Print and shaded views of the part. All mm, measured from the part's lowest x, y and z. A direction names the side the tool comes from. Coordinates: 2 decimals unless noted, no trailing zeros. Loops run counter-clockwise (first coordinate to the right, second up) from the corner with the lowest first, then second, coordinate; pieces in that order, holes last.
1) Pin check, flat tips, straight feed: pin 1 Ø1.7 at (y, z) = (16.5, 6.5) entering from +X; pin 2 Ø1.5 at (x, y) = (13, 12) entering from +Z; pin 3 Ø4.5 at (x, z) = (11, 11.5) entering from +Y; pin 4 Ø3 at (y, z) = (17.5, 6.5) entering from -X. Stop position of each tip, or through.
2) Which spindle directions (+Z, -Z, +X, -X, +Y, -Y) get a long thin tool onto all of the face, cutting with end or side? Do the marked faces 1, 2 and 3. Say none if no direction does.
3) Saw through at B-B, the plane x = 2. Write the cut outline in (y, z) (1 decimal).
4) Saw through at A-A, the plane y = 16.75. Write the cut outline in (x, z) (1 decimal), and give its area (3 significant figures).
5) Saw through at C-C, the plane z = 3.75. Write the cut outline in (x, y) (1 decimal).
6) Wall check: line 1 along Y through (x, z) = (2, 11.25); line 2 along X through (y, z) = (14, 7.5); line 3 along Y through (x, z) = (9, 1.25). Give the ranges that are in metal, low to high.
7) Saw through at D-D, the plane y = 10.75. Write the cut outline in (x, z), and give its area (3 significant figures).
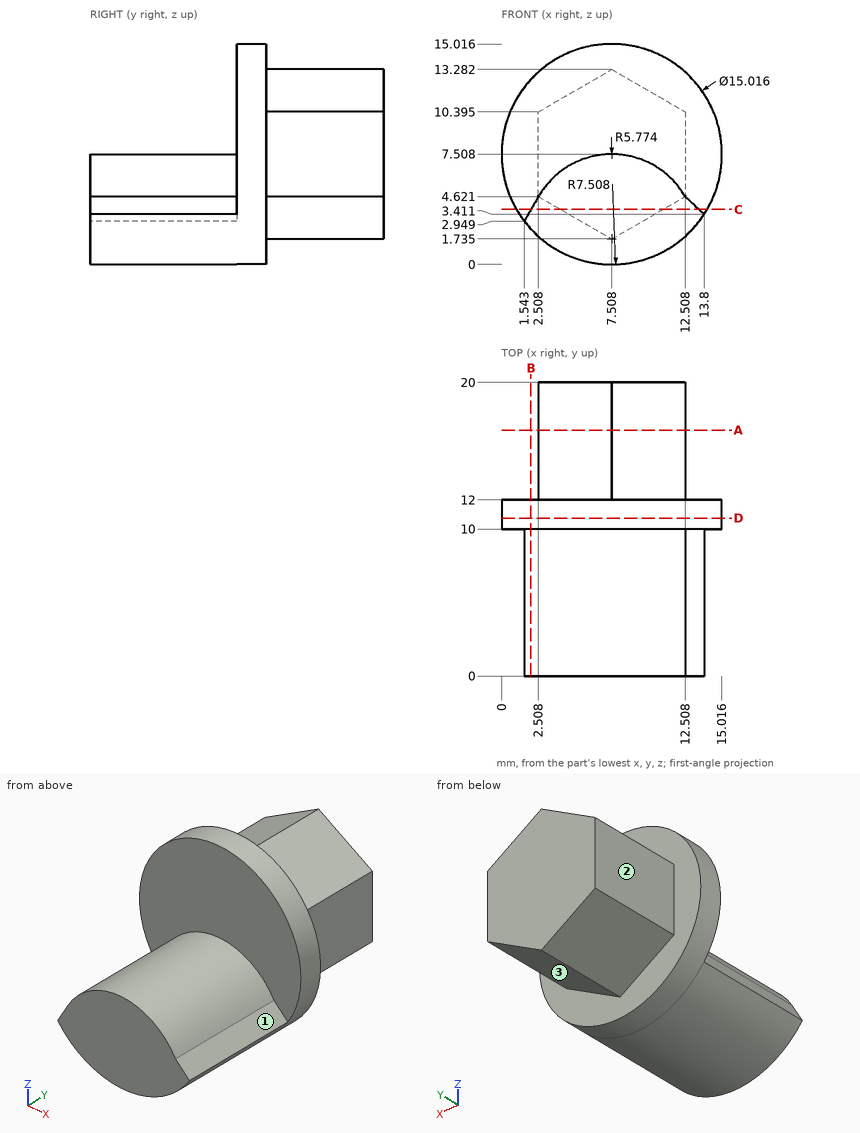
Data:
1. pin 1: stops at x = 12.51
1. pin 2: stops at z = 13.33
1. pin 3: stops at y = 20
1. pin 4: stops at x = 2.51
2. face 1: +Z, +X, -Y
2. face 2: +Z, -Z, -X, +Y
2. face 3: -Z, +X, +Y
3. outline: (0, 2.4) - (12, 2.4) - (12, 12.6) - (10, 12.6) - (10, 3.7) - (0, 3.7) - close
4. outline: (2.5, 4.6) - (7.5, 1.7) - (12.5, 4.6) - (12.5, 10.4) - (7.5, 13.3) - (2.5, 10.4) - close
4. area: 86.6 mm2
5. outline: (1, 10) - (2, 10) - (2, 0) - (13.4, 0) - (13.4, 10) - (14, 10) - (14, 12) - (11, 12) - (11, 20) - (4, 20) - (4, 12) - (1, 12) - close
6. line 1: y = 10 to 12
6. line 2: x = 2.51 to 12.51
6. line 3: y = 0 to 12
7. outline: circle Ø15.02 at (7.51, 7.51)
7. area: 177 mm2
